Can you work these out from the model? Positions are in its coordinate system, mm. Give positions to 0.01 mm unless a question says otherwise; leave off trailing zeros. Order: outer loops, then holes, each group sorted by start corner. A loop starts at its lowest first (then second) coordinate and runs counter-clockwise, first axis right, second up.
Item 1: I want a section at B-B, the plane z = 1. Count the separate pieces of the cut face and the enclosed holes in it, then the cut area to 3 significant figures.
Item 2: If I drill on line 1 along Y through (x, z) = (170, 1); line 2 along X through (y, z) = (123.5, 4.5); line 3 along X through (y, z) = (39, 1.75), over which ranges is the centre line in solid material (lowest first)?
Item 3: I want a section at A-A, the plane y = 53. Write out the boundary of the cut face in (x, z).
Item 4: I'm going to push flat-ended pins straight in: pin 1 Ø1.5 at (y, z) = (127, 1) entering from +X; pin 2 Ø1.6 at (x, y) = (154.5, 129) entering from +Z; pin 3 Ø1 at (x, z) = (146, 5) entering from +Y. Where does each tip first touch, or does it pass through?
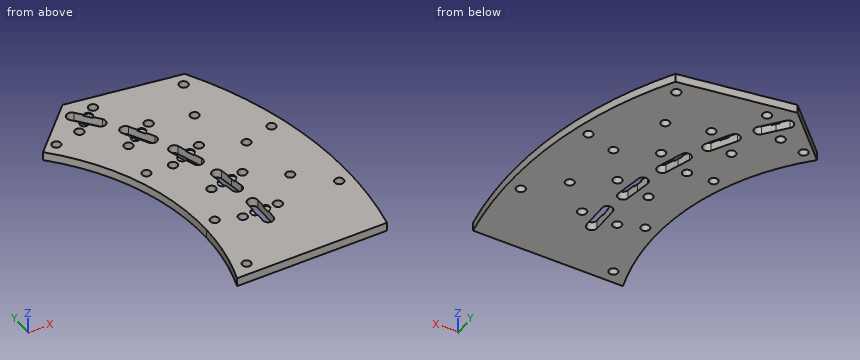
```python
from build123d import *

# Parameters (mm, degrees)
SKETCH1_R           = 3.175
SKETCH1_R_2         = 3.2639
BOSS_EXTRUDE1_DEPTH = 6.35
SKETCH2_R           = 3.175
CUT_EXTRUDE1_DEPTH  = 0.79375


with BuildPart() as part:
    # Sketch1 → Boss-Extrude1 (new body)
    with BuildSketch(Plane.XY):
        with BuildLine():
            Line((159.591131024, -50.8), (268.282803213, -50.8))
            ThreePointArc((268.282803213, -50.8), (268.798556268, 47.996235774), (234.123018172, 140.508771477))
            Line((234.123018172, 140.508771477), (152.715190262, 152.715190262))
            Line((152.715190262, 152.715190262), (118.427127597, 118.427127597))
            ThreePointArc((118.427127597, 118.427127597), (154.732498954, 64.092299607), (167.48125, 0))
            ThreePointArc((167.48125, 0), (165.496965553, -25.70454229), (159.591131024, -50.8))
        make_face()
        with Locations((176.898422575, 6.177429038)):
            Circle(SKETCH1_R, mode=Mode.SUBTRACT)
        with Locations((129.454176147, 120.717972221)):
            Circle(SKETCH1_R, mode=Mode.SUBTRACT)
        with Locations((163.532451502, 67.7373593)):
            Circle(SKETCH1_R, mode=Mode.SUBTRACT)
        with Locations((172.12665951, -41.275)):
            Circle(SKETCH1_R, mode=Mode.SUBTRACT)
        with Locations((193.675, 0)):
            Circle(SKETCH1_R_2, mode=Mode.SUBTRACT)
        with Locations((219.075, 0)):
            Circle(SKETCH1_R_2, mode=Mode.SUBTRACT)
        with Locations((215.746758491, 38.041974522)):
            Circle(SKETCH1_R_2, mode=Mode.SUBTRACT)
        with Locations((190.732641565, 33.63131081)):
            Circle(SKETCH1_R_2, mode=Mode.SUBTRACT)
        with Locations((205.863160899, 74.928062899)):
            Circle(SKETCH1_R_2, mode=Mode.SUBTRACT)
        with Locations((181.994968331, 66.240751259)):
            Circle(SKETCH1_R_2, mode=Mode.SUBTRACT)
        with Locations((189.724515334, 109.5375)):
            Circle(SKETCH1_R_2, mode=Mode.SUBTRACT)
        with Locations((167.727470078, 96.8375)):
            Circle(SKETCH1_R_2, mode=Mode.SUBTRACT)
        with Locations((167.821186376, 140.818695592)):
            Circle(SKETCH1_R_2, mode=Mode.SUBTRACT)
        with Locations((148.363657521, 124.491890306)):
            Circle(SKETCH1_R_2, mode=Mode.SUBTRACT)
        with Locations((263.525, 0)):
            Circle(SKETCH1_R_2, mode=Mode.SUBTRACT)
        with Locations((254.545603373, 68.205288861)):
            Circle(SKETCH1_R_2, mode=Mode.SUBTRACT)
        with Locations((228.219344532, 131.7625)):
            Circle(SKETCH1_R_2, mode=Mode.SUBTRACT)
        with Locations((240.38178065, 21.030680725)):
            Circle(SKETCH1_R, mode=Mode.SUBTRACT)
        with Locations((233.077901884, 62.453035583)):
            Circle(SKETCH1_R, mode=Mode.SUBTRACT)
        with Locations((218.692069012, 101.977786558)):
            Circle(SKETCH1_R, mode=Mode.SUBTRACT)
        with BuildLine():
            Line((202.565, 0), (202.565, 9.525))
            ThreePointArc((202.565, 9.525), (206.375, 13.335), (210.185, 9.525))
            Line((210.185, 9.525), (210.185, 0))
            Line((210.185, 0), (210.185, -9.525))
            ThreePointArc((210.185, -9.525), (206.375, -13.335), (202.565, -9.525))
            Line((202.565, -9.525), (202.565, 0))
        make_face(mode=Mode.SUBTRACT)
        with BuildLine():
            Line((199.487582489, 35.175043109), (201.141581381, 25.794749262))
            ThreePointArc((201.141581381, 25.794749262), (205.555298477, 22.70423128), (208.645816459, 27.117948375))
            Line((208.645816459, 27.117948375), (206.991817567, 36.498242223))
            Line((206.991817567, 36.498242223), (205.337818675, 45.87853607))
            ThreePointArc((205.337818675, 45.87853607), (200.924101579, 48.969054052), (197.833583597, 44.555336957))
            Line((197.833583597, 44.555336957), (199.487582489, 35.175043109))
        make_face(mode=Mode.SUBTRACT)
        with BuildLine():
            Line((190.348835729, 69.281310333), (193.606577595, 60.33073812))
            ThreePointArc((193.606577595, 60.33073812), (198.489903226, 58.053605981), (200.767035365, 62.936931612))
            Line((200.767035365, 62.936931612), (197.5092935, 71.887503825))
            Line((197.5092935, 71.887503825), (194.251551635, 80.838076038))
            ThreePointArc((194.251551635, 80.838076038), (189.368226003, 83.115208177), (187.091093864, 78.231882546))
            Line((187.091093864, 78.231882546), (190.348835729, 69.281310333))
        make_face(mode=Mode.SUBTRACT)
        with BuildLine():
            Line((175.426435918, 101.2825), (180.188935918, 93.033608029))
            ThreePointArc((180.188935918, 93.033608029), (185.393492706, 91.639051241), (186.788049494, 96.843608029))
            Line((186.788049494, 96.843608029), (182.025549494, 105.0925))
            Line((182.025549494, 105.0925), (177.263049494, 113.341391971))
            ThreePointArc((177.263049494, 113.341391971), (172.058492706, 114.735948759), (170.663935918, 109.531391971))
            Line((170.663935918, 109.531391971), (175.426435918, 101.2825))
        make_face(mode=Mode.SUBTRACT)
        with BuildLine():
            Line((155.17379262, 130.206272156), (161.296344603, 122.909698835))
            ThreePointArc((161.296344603, 122.909698835), (166.663994724, 122.4400903), (167.133603259, 127.807740421))
            Line((167.133603259, 127.807740421), (161.011051277, 135.104313742))
            Line((161.011051277, 135.104313742), (154.888499295, 142.400887063))
            ThreePointArc((154.888499295, 142.400887063), (149.520849174, 142.870495598), (149.051240638, 137.502845477))
            Line((149.051240638, 137.502845477), (155.17379262, 130.206272156))
        make_face(mode=Mode.SUBTRACT)
    extrude(amount=BOSS_EXTRUDE1_DEPTH)

    # Sketch2 → Cut-Extrude1 (cut)
    with BuildSketch(Plane.XY.offset(6.35)):
        with Locations((202.565, 0)):
            Circle(SKETCH2_R)
        with Locations((210.185, 0)):
            Circle(SKETCH2_R)
        with Locations((199.487582489, 35.175043109)):
            Circle(SKETCH2_R)
        with Locations((206.991817567, 36.498242223)):
            Circle(SKETCH2_R)
        with Locations((190.348835729, 69.281310333)):
            Circle(SKETCH2_R)
        with Locations((197.5092935, 71.887503825)):
            Circle(SKETCH2_R)
        with Locations((175.426435918, 101.2825)):
            Circle(SKETCH2_R)
        with Locations((182.025549494, 105.0925)):
            Circle(SKETCH2_R)
        with Locations((155.17379262, 130.206272156)):
            Circle(SKETCH2_R)
        with Locations((161.011051277, 135.104313742)):
            Circle(SKETCH2_R)
    extrude(amount=-CUT_EXTRUDE1_DEPTH, mode=Mode.SUBTRACT)


solid = part.part
```
Results list:
1. separate pieces: 1
1. enclosed holes: 25
1. area: 20,100 mm2
2. line 1: y = -50.8 to -43.63, -38.92 to 94.49, 99.18 to 138.39, 143.25 to 150.12
2. line 2: x = 123.5 to 127.92, 130.98 to 145.25, 151.47 to 160.8, 167.54 to 243.52
2. line 3: x = 162.88 to 198.81, 206.55 to 212.63, 218.87 to 270.25
3. outline: (158.87, 0) - (267.86, 0) - (267.86, 6.35) - (158.87, 6.35) - close
4. pin 1: stops at x = 242.11
4. pin 2: stops at z = 5.56
4. pin 3: stops at y = 146.5
